from build123d import *

# Parameters (mm, degrees)
SCHNITT_LINEAR_AUSTRAGEN1_DEPTH = 2.7
SKIZZE3_W                       = 7
SKIZZE3_H                       = 2.1
SKIZZE4_W                       = 3.9
SKIZZE4_H                       = 0.5


with BuildPart() as part:
    # Skizze1 → Rotation1 (revolve)
    with BuildSketch(Plane.XY):
        Polygon((-4, 0), (7, 0), (7, 2), (0, 2), (0, 3.6), (-4, 3.6), align=None)
    revolve(axis=Axis((-29.304407472, 0, 0), (1, 0, 0)))

    # Skizze2 → Schnitt-Linear austragen1 (cut)
    with BuildSketch(Plane.ZY.offset(4)):
        Polygon((0, 1.732050808), (-1.5, 0.866025404), (-1.5, -0.866025404), (0, -1.732050808), (1.5, -0.866025404), (1.5, 0.866025404), align=None)
    extrude(amount=-SCHNITT_LINEAR_AUSTRAGEN1_DEPTH, mode=Mode.SUBTRACT)

    # Skizze3 → Schnitt-Rotation1 (revolve, cut)
    with BuildSketch(Plane.XY):
        with Locations((3.5, 2.55)):
            Rectangle(SKIZZE3_W, SKIZZE3_H)
    revolve(axis=Axis((-0.757628828, 0, 0), (1, 0, 0)), mode=Mode.SUBTRACT)

    # Skizze4 → Schnitt-Rotation2 (revolve, cut)
    with BuildSketch(Plane.XY):
        with Locations((5.05, 1.25)):
            Rectangle(SKIZZE4_W, SKIZZE4_H)
    revolve(axis=Axis((0, 0, 0), (1, 0, 0)), mode=Mode.SUBTRACT)

    # Skizze6 → Schnitt-Rotation3 (revolve, cut)
    with BuildSketch(Plane.XY):
        Polygon((-2.7, 3), (0, 3), (0, 3.6), (-4, 3.6), (-4, 0), (-2.7, 0), align=None)
    revolve(axis=Axis((-4.405632507, 0, 0), (1, 0, 0)), mode=Mode.SUBTRACT)


solid = part.part
Can you work these out from the model? Positions are in its coordinate system, mm. A direction names the side the tool comes from. Coordinates: 2 decimals unless noted, no trailing zeros. Write each loop counter-clockwise with the first axis right and the second up, starting at its lowest first coordinate (ties: lowest second). Pieces come first, ordered by that corner, then holes. Notation, with made-up numbers: M 61.25,18 L 107.25,18 A17 ccw 107.25,41 Z; hole C -38,35 d3. An arc over 180 degrees is marked long. Use one line per item in the form item = value.
Q1. If we section it at D-D (x = 1.5): Write out the boundary of the cut face in (y, z).
Model answer:
outline = C 0,0 d3
Q2. For faces 1 (the flat face through (0, -1.3, -1.3)), 2 (the flat face through (-2.7, -1.3, -1.3)), 3 (the flat face through (-2.01, 1.293, 0.76)), which set-ups out of +Z, -Z, +X, -X, +Y, -Y let a thin tool reach every point of the face, with its end or its side?
Model answer:
face_1 = +X
face_2 = +Z, -Z, -X, +Y, -Y
face_3 = -X
Q3. If we section it at A-A (x = -1.5): Write out the boundary of the cut face in (y, z).
Model answer:
outline = C 0,0 d6; hole M -1.73,0 L -0.87,-1.5 L 0.87,-1.5 L 1.73,0 L 0.87,1.5 L -0.87,1.5 Z
Q4. If we section it at C-C (z = -0.5): Write out the boundary of the cut face in (x, y).
Model answer:
outline = M -2.7,-2.96 L 0,-2.96 L 0,-1.41 L 3.1,-1.41 L 3.1,-0.87 L 7,-0.87 L 7,0.87 L 3.1,0.87 L 3.1,1.41 L 0,1.41 L 0,2.96 L -2.7,2.96 L -2.7,1.44 L -1.3,1.44 L -1.3,-1.44 L -2.7,-1.44 Z
Q5. We'd pull the mould along Z, two halves only. Please class faces 4 (the flat face through (-2.01, -1.305, 0.74)), 5 (the cylindrical face through (1.6, -1.2, -0.9)), 6 (the flat face through (7, 0, 0)): +Z half, -Z half, draft (parallel to the pull), parting line (faces both ways), or undercut.
Model answer:
face_4 = undercut
face_5 = parting line
face_6 = draft
Q6. For P1, Ø2, axis at x = 3.5, y = 1, coming from the +Z side; P2, Ø1.1, axis at x = -2.5, y = 0.5, coming from the +Z side; P3, Ø1.5, axis at x = 1, y = 0, coming from the -Z side; P4, Ø3, axis at y = 0.5, z = -2.5, coming from the +X side, each with a flat end and sliding along its axis, tell me the tip position at first contact or that it passes through.
Model answer:
P1 = 1.5
P2 = 3
P3 = -1.5
P4 = 3.1
Q7. I need wall thicknesses on line 1 along X through (y, z) = (-1.55, 0.45); line 2 along X through (y, z) = (-1.2, 0.8); line 3 along Y through (x, z) = (6, -0.05). Which ranges of each line are inside material? Lowest first, please. Write a range as from..to.
Model answer:
line_1 = -2.7..0
line_2 = -1.3..3.1
line_3 = -1..1
Q8. If we section it at B-B (y = 0): Write out the boundary of the cut face in (x, z).
Model answer:
outline = M -2.7,-3 L 0,-3 L 0,-1.5 L 3.1,-1.5 L 3.1,-1 L 7,-1 L 7,1 L 3.1,1 L 3.1,1.5 L 0,1.5 L 0,3 L -2.7,3 L -2.7,1.5 L -1.3,1.5 L -1.3,-1.5 L -2.7,-1.5 Z
